Design review of the part built by this model. Coordinates are the model's own, in mm. A direction names the side the tool comes from. Round coordinates to 2 decimals unless told otherwise and drop trailing zeros. Write each loop counter-clockwise with the first axis right and the second up, starting at its lowest first coordinate (ties: lowest second). Pieces come first, ordered by that corner, then holes. Notation, with made-up numbers: (-16.5, 50.5) - (6.5, 50.5) arc R21 cw to (6.5, 75.5) - close; hole circle Ø2 at (72.5, -10). An arc over 180 degrees is marked (long way). Use one line per item in the form item = value.
```python
from build123d import *

# Parameters (mm, degrees)
SKETCH_W     = 80
SKETCH_H     = 130
PAD_DEPTH    = 18
THICKNESS_T  = -1
POCKET_DEPTH = 130.001
FILLET_R     = 2


with BuildPart() as part:
    # Sketch → Pad (new body)
    with BuildSketch(Plane.XY):
        Rectangle(SKETCH_W, SKETCH_H)
    extrude(amount=PAD_DEPTH)

    # Thickness
    thickness_openings = [part.faces().sort_by_distance(p)[0] for p in [
        (0, 65, 9),
    ]]
    offset(amount=THICKNESS_T, openings=thickness_openings)

    # Sketch001 (on Face2 of Thickness) → Pocket (cut, through all)
    with BuildSketch(Plane.XZ.offset(65)):
        with BuildLine():
            Line((-26, 15.5), (26, 15.5))
            ThreePointArc((29, 12.5), (28.12132, 14.62132), (26, 15.5))
            Line((29, 12.5), (29, 5.5))
            ThreePointArc((26, 2.5), (28.12132, 3.37868), (29, 5.5))
            Line((26, 2.5), (-26, 2.5))
            ThreePointArc((-29, 5.5), (-28.12132, 3.37868), (-26, 2.5))
            Line((-29, 5.5), (-29, 12.5))
            ThreePointArc((-26, 15.5), (-28.12132, 14.62132), (-29, 12.5))
        make_face()
    extrude(amount=-POCKET_DEPTH, mode=Mode.SUBTRACT)

    # Fillet
    fillet_edges = [part.edges().sort_by_distance(p)[0] for p in [
        (-40, 0, 0),
        (40, 0, 0),
        (-40, 0, 18),
        (0, -65, 18),
        (-40, -65, 9),
        (0, -65, 0),
        (40, -65, 9),
        (40, 0, 18),
    ]]
    fillet(fillet_edges, radius=FILLET_R)


solid = part.part
```
Q1. For P1, Ø0.8, axis at x = 3.5, y = -64.5, coming from the +Z side; P2, Ø2, axis at x = -12.5, z = 14, coming from the +Y side; P3, Ø0.5, axis at y = -64.5, z = 10.5, coming from the +X side; P4, Ø0.8, axis at y = -64.5, z = 10, coming from the -X side, all flat-tipped, find the tip position at first contact; note any pin that passes through.
Calculated:
P1 = 17.67
P2 = through
P3 = 39.56
P4 = -39.67
Q2. To check wall thickness, follow line 1 along Z through (x, y) = (21, -3.5); line 2 along X through (y, z) = (-39.5, 6.5); line 3 along Y through (x, z) = (-34, 10.75). State the ranges of each line that lie inside material, in increasing order. Write a range as from..to.
Calculated:
line_1 = 0..1, 17..18
line_2 = -40..-39, 39..40
line_3 = -65..-64
Q3. Draft analysis for pull direction Z (two halves, no side actions). For faces 1 (the flat face through (-1, 2, 18)), 2 (the flat face through (39, 0, 9)), 3 (the flat face through (-0.2, -65, 15.7)), state which applies: released by +Z, released by -Z, zero draft, split by the parting line, or undercut.
Calculated:
face_1 = released by +Z
face_2 = undercut
face_3 = zero draft
Q4. We need section B-B on y = 32. Write out the cut boundary in (x, z).
Calculated:
outline = (-40, 2) arc R2 ccw to (-38, 0) - (38, 0) arc R2 ccw to (40, 2) - (40, 16) arc R2 ccw to (38, 18) - (-38, 18) arc R2 ccw to (-40, 16) - close; hole (-39, 1) - (39, 1) - (39, 17) - (-39, 17) - close
Q5. We need section A-A on z = 8.25. Write out the cut boundary in (x, y), then the cut area to 3 significant figures.
Calculated:
outline = (-40, -63) arc R2 ccw to (-38, -65) - (-29, -65) - (-29, -64) - (-39, -64) - (-39, 65) - (-40, 65) - close; (29, -65) - (38, -65) arc R2 ccw to (40, -63) - (40, 65) - (39, 65) - (39, -64) - (29, -64) - close
area = 278 mm2
Q6. Machinability: for faces 4 (the flat face through (-1, 1, 1)), 5 (the cylindrical face through (-28.14, -64.51, 3.4)), 6 (the flat face through (-40, 0, 9)), which of the approach directions +Z, -Z, +X, -X, +Y, -Y give a long, thin tool a straight path to every point of the face, cutting with its end or side? Answer none if there is none.
Calculated:
face_4 = +Y
face_5 = +Y, -Y
face_6 = +Z, -Z, -X, +Y, -Y
Q7. We need section C-C on x = 32. Write out the cut boundary in (y, z), then the cut area to 3 significant figures.
Calculated:
outline = (-65, 2) arc R2 ccw to (-63, 0) - (65, 0) - (65, 1) - (-64, 1) - (-64, 17) - (65, 17) - (65, 18) - (-63, 18) arc R2 ccw to (-65, 16) - close
area = 274 mm2
Q8. We need section D-D on x = -20.5. Write out the cut boundary in (y, z).
Calculated:
outline = (-65, 2) arc R2 ccw to (-63, 0) - (65, 0) - (65, 1) - (-64, 1) - (-64, 2.5) - (-65, 2.5) - close; (-65, 15.5) - (-64, 15.5) - (-64, 17) - (65, 17) - (65, 18) - (-63, 18) arc R2 ccw to (-65, 16) - close
